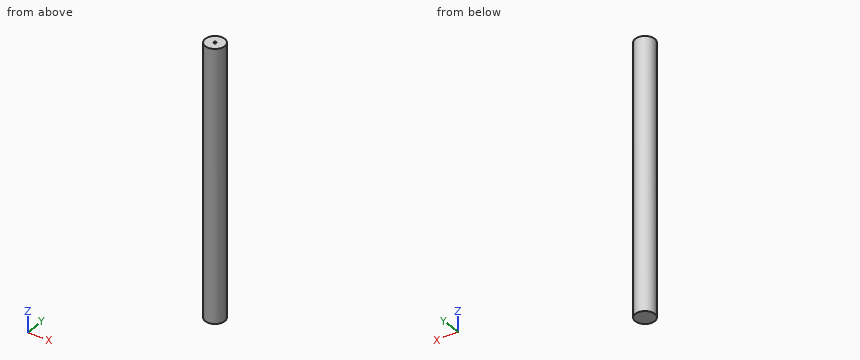
```python
from build123d import *

# Parameters (mm, degrees)
IZIM1_R                     = 4
Y_KSEKLIK_EKSTR_ZYON1_DEPTH = 110
IZIM2_R                     = 0.5
KES_EKSTR_ZYON1_DEPTH       = 5
RADYUS1_R                   = 0.1


with BuildPart() as part:
    # Çizim1 → Yükseklik-Ekstrüzyon1 (new body)
    with BuildSketch(Plane.XY):
        Circle(IZIM1_R)
    extrude(amount=Y_KSEKLIK_EKSTR_ZYON1_DEPTH)

    # Çizim2 → Kes-Ekstrüzyon1 (cut)
    with BuildSketch(Plane.XY.offset(110)):
        Circle(IZIM2_R)
    extrude(amount=-KES_EKSTR_ZYON1_DEPTH, mode=Mode.SUBTRACT)

    # Radyus1
    radyus1_edges = [part.edges().sort_by_distance(p)[0] for p in [
        (-0.5, 0, 110),
    ]]
    fillet(radyus1_edges, radius=RADYUS1_R)


solid = part.part
```
Geometry check sheet. Reference: the model listing, model coordinates, mm. Give positions to 0.01 mm unless a question says otherwise; leave off trailing zeros. Order: outer loops, then holes, each group sorted by start corner. A loop starts at its lowest first (then second) coordinate and runs counter-clockwise, first axis right, second up. Notation, with made-up numbers: (69.25, 20) - (73.25, 20) arc R6 ccw to (73.25, 27) - close; hole circle Ø8 at (81.25, 49.25). An arc over 180 degrees is marked (long way). Write item = value, one per line. Start each with the question number.
1) Gauge pin test, flat ends, axial feed: pin 1 Ø3 at (x, z) = (2.5, 44.5) entering from +Y; pin 2 Ø1 at (x, z) = (-3, 73.5) entering from -Y; pin 3 Ø2 at (y, z) = (1.5, 53.5) entering from -X. Record the tip position at first contact, or that the pin passes through.
2) Section check A-A (z = 59). Enter the section's corners in (x, y), then the cut area to 3 significant figures.
3) Section check B-B (x = -1.5). Enter the section's corners in (y, z).
4) Scan lines: L1, parallel to Y at x = 0, z = 107.7; L2, parallel to X at y = 0.25, z = 65.5; L3, parallel to X at y = -1.5, z = 18.5. Record each from-to range of solid material in increasing order.
Geometry check:
q1.pin_1 = 3.87
q1.pin_2 = -3.12
q1.pin_3 = -3.97
q2.outline = circle Ø8 at (0, 0)
q2.area = 50.3 mm2
q3.outline = (-3.71, 0) - (3.71, 0) - (3.71, 110) - (-3.71, 110) - close
q4.L1 = -4 to -0.5, 0.5 to 4
q4.L2 = -3.99 to 3.99
q4.L3 = -3.71 to 3.71
